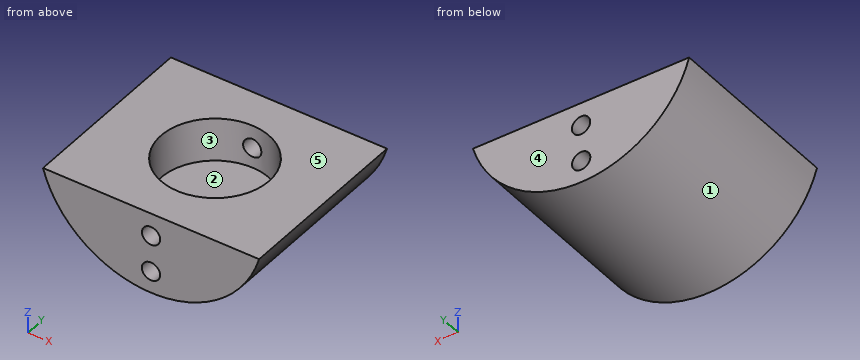
```python
from build123d import *

# Parameters (mm, degrees)
F1_DEPTH      = 25.4
F1_DEPTH_BACK = 25.4
F2_R          = 15
F3_DEPTH      = 12
F5_R          = 2.54
F6_DEPTH      = 127


with BuildPart() as f1:
    # F0 (on Front) → F1 (new body, two sides)
    with BuildSketch(Plane.XZ) as f1_sk:
        with BuildLine():
            Line((30, 0), (-30, 0))
            ThreePointArc((-30, 0), (0, -22.597278), (30, 0))
        make_face()
    extrude(amount=F1_DEPTH)
    extrude(f1_sk.sketch, amount=-F1_DEPTH_BACK)

    # F2 (on face) → F3 (cut)
    with BuildSketch(Plane.XY):
        Circle(F2_R)
    extrude(amount=-F3_DEPTH, mode=Mode.SUBTRACT)

    # F5 (on face) → F6 (cut)
    with BuildSketch(Plane.XZ.offset(25.4)):
        with Locations((0, -6.35)):
            Circle(F5_R)
        with Locations((-0.024882, -16.51)):
            Circle(F5_R)
    extrude(amount=-F6_DEPTH, mode=Mode.SUBTRACT)


solid = f1.part
```
Geometry: final body of the model. Coordinates: model frame, mm. Face numbers are marked on the shaded views. A direction names the side the tool comes from. Give positions to 0.01 mm unless a question says otherwise; leave off trailing zeros. Write each loop counter-clockwise with the first axis right and the second up, starting at its lowest first coordinate (ties: lowest second). Pieces come first, ordered by that corner, then holes.
1. Draft query along Y for the marked faces 3, 4 and 5. Return one class per face: released by +Y, released by -Y, zero draft, split by the parting line, or undercut.
2. Section query C-C, the plane z = -16.51. Return loops of the section in (x, y), then the cut area to 3 significant figures.
3. Section query A-A, the plane y = 0. Return loops of the section in (x, z), then the cut area to 3 significant figures.
4. Reachability of the marked faces 1 and 2 from +Z, -Z, +X, -X, +Y, -Y: full face, straight path, thin tool, end or side. Return the list, or none.
5. Section query B-B, the plane x = 0. Return loops of the section in (y, z), then the cut area to 3 significant figures.
6. Line query: probe 1 along Z at (x, y) = (0, -21.25); probe 2 along Y at (x, z) = (0, -3.5); probe 3 along Y at (x, z) = (-2.5, -5). Output: solid intervals per line, ascending.
7. Section query D-D, the plane x = 10.5. Return loops of the section in (y, z), then the cut area to 3 significant figures.
8. Pin query (flat end, axial travel): P1, Ø10, axis at x = -12, y = 6.5, coming from the -Z side; P2, Ø6.5, axis at x = -0.02, z = -16.51, coming from the -Y side; P3, Ø6, axis at y = -17, z = -16.5, coming from the -X side; P4, Ø10, axis at y = 14, z = -11, coming from the -X side. Return the tip coordinate at first contact, or that it passes through.
Computed:
1. face 3: undercut
1. face 4: released by +Y
1. face 5: zero draft
2. outline: (-18.52, -25.4) - (-2.56, -25.4) - (-2.56, 25.4) - (-18.52, 25.4) - close; (2.52, -25.4) - (18.52, -25.4) - (18.52, 25.4) - (2.52, 25.4) - close
2. area: 1,620 mm2
3. outline: (-30, 0) arc R31.21 ccw to (30, 0) - (15, 0) - (15, -12) - (-15, -12) - (-15, 0) - close; hole circle Ø5.08 at (-0.02, -16.51)
3. area: 619 mm2
4. face 1: -Z, +Y, -Y
4. face 2: +Z
5. outline: (-25.4, -22.6) - (25.4, -22.6) - (25.4, -19.05) - (-25.4, -19.05) - close; (-25.4, -13.97) - (25.4, -13.97) - (25.4, -8.89) - (15, -8.89) - (15, -12) - (-15, -12) - (-15, -8.89) - (-25.4, -8.89) - close; (-25.4, -3.81) - (-15, -3.81) - (-15, 0) - (-25.4, 0) - close; (15, -3.81) - (25.4, -3.81) - (25.4, 0) - (15, 0) - close
5. area: 424 mm2
6. probe 1: z = -22.6 to -19.05, -13.97 to -8.89, -3.81 to 0
6. probe 2: y = -25.4 to -15, 15 to 25.4
6. probe 3: y = -25.4 to -14.79, 14.79 to 25.4
7. outline: (-25.4, -20.78) - (25.4, -20.78) - (25.4, 0) - (10.71, 0) - (10.71, -12) - (-10.71, -12) - (-10.71, 0) - (-25.4, 0) - close
7. area: 798 mm2
8. P1: stops at z = -21.8
8. P2: stops at y = -25.4
8. P3: stops at x = -22.03
8. P4: stops at x = -27.58
